Check sheet for the modelled part. Datum: model origin and axes. Units: mm. A direction names the side the tool comes from. Give positions to 0.01 mm unless a question says otherwise; leave off trailing zeros. Write each loop counter-clockwise with the first axis right and the second up, starting at its lowest first coordinate (ties: lowest second). Pieces come first, ordered by that corner, then holes. Notation, with made-up numbers: (-27, 13.25) -> (10, 13.25) arc R31 cw to (10, 42.25) -> close; hole circle Ø5 at (-38, 39). An arc over 180 degrees is marked (long way). Answer as a JSON object with one key per item and string values.
from build123d import *

# Parameters (mm, degrees)
F1_R     = 70
F4_DEPTH = 80
F5_R     = 62
F6_DEPTH = 85
F7_W     = 435.71645
F7_H     = 77.360585
F8_DEPTH = 80


with BuildPart() as f3:
    # F3: sweep along a path in F0
    with BuildLine(Plane.XZ) as f3_path:
        Line((64, 0), (64, 194))
        ThreePointArc((64, 194), (-68, 326), (-200, 194))
        Line((-200, 194), (-200, 0))
    # F1 (on Top) → F3 (sweep)
    with BuildSketch(Plane.XY):
        with Locations((64, 0)):
            Circle(F1_R)
    sweep(path=f3_path.line)

    # F2 (on Front) → F4 (join)
    with BuildSketch(Plane.XZ):
        with BuildLine():
            Line((-270, 194), (134, 194))
            ThreePointArc((134, 194), (-68, 396), (-270, 194))
        make_face()
        with BuildLine():
            ThreePointArc((-270, 194), (-68, -8), (134, 194))
            Line((134, 194), (-270, 194))
        make_face()
        with BuildLine():
            Line((134, -18.768641), (134, 194))
            ThreePointArc((134, 194), (-68, -8), (-270, 194))
            Line((-270, 194), (-270, -18.768641))
            Line((-270, -18.768641), (134, -18.768641))
        make_face()
    extrude(amount=-F4_DEPTH)

    # F5 (on Front) → F6 (cut)
    with BuildSketch(Plane.XZ):
        with Locations((-68, 194)):
            Circle(F5_R)
    extrude(amount=-F6_DEPTH, mode=Mode.SUBTRACT)

    # F7 (on Front) → F8 (cut)
    with BuildSketch(Plane.XZ):
        with Locations((-63.542128, -38.680293)):
            Rectangle(F7_W, F7_H)
    extrude(amount=-F8_DEPTH, mode=Mode.SUBTRACT)


solid = f3.part
1. Mould release check, pull along Z, two halves, no side actions. Record for faces 3 (the face through (62.461, -69.983, 98.358)), 4 (the face through (-71, 39, 0)), 5 (the face through (-76.071, 39.44, 255.472)), 6 (the face through (-63.56, 39.44, 395.95)): released by +Z, released by -Z, zero draft, split by the parting line, or undercut.
Determined:
{"face 3": "zero draft", "face 4": "released by -Z", "face 5": "undercut", "face 6": "released by +Z"}
2. Scan lines: L1, parallel to Z at x = -68, y = 49; L2, parallel to X at y = -0.5, z = 179; L3, parallel to Y at x = -1, z = 312. Record each from-to range of solid material in increasing order. Write a range as [from, to].
Determined:
{"L1": "[0, 132], [256, 396]", "L2": "[-270, -130], [-6, 134]", "L3": "[-69.9, 80]"}
3. Sectioned sample at D-D, the plane y = -30. Enter the section's corners in (x, z).
Determined:
{"outline": "(-263.25, 0) -> (-136.75, 0) -> (-136.75, 194) arc R68.75 cw to (0.75, 194) -> (0.75, 0) -> (127.25, 0) -> (127.25, 194) arc R195.25 ccw to (-263.25, 194) -> close"}
4. Access from +Z, -Z, +X, -X, +Y, -Y to the whole of each face (thin tool, end or side, straight path). Record for faces 1 (the face through (-69, 0, 69)), 2 (the face through (-71, 80, 113)).
Determined:
{"face 1": "-Z, -Y", "face 2": "+Z, -Z, +X, -X, +Y"}
5. Go/stop test with flat-tipped pins: P1, Ø4, axis at x = -228.5, z = 108.5, coming from the -Y side; P2, Ø1.5, axis at y = 33, z = 298, coming from the +X side; P3, Ø10, axis at x = 53.5, z = 327, coming from the -Y side. Record where each tip stops, or that it passes through.
Determined:
{"P1": "y = -64.79", "P2": "x = 105.62", "P3": "y = -55.12"}
6. Sectioned sample at A-A, the plane x = -68. Enter the section's corners in (y, z), plus the area to 3 significant figures.
Determined:
{"outline": "(0, 0) -> (80, 0) -> (80, 132) -> (0, 132) -> close; (0, 256) -> (80, 256) -> (80, 396) -> (0, 396) arc R70 ccw to start", "area": "29,500 mm^2"}
7. Sectioned sample at B-B, the plane y = 17. Enter the section's corners in (x, z).
Determined:
{"outline": "(-270, 0) -> (134, 0) -> (134, 194) arc R202 ccw to (-270, 194) -> close; hole circle Ø124 at (-68, 194)"}
8. Sectioned sample at C-C, the plane z = 59. Enter the section's corners in (x, y), plus the area to 3 significant figures.
Determined:
{"outline": "(-270, 0) arc R70 ccw to (-130, 0) -> (-6, 0) arc R70 ccw to (134, 0) -> (134, 80) -> (-270, 80) -> close", "area": "47,700 mm^2"}
